Model file for the job. Use its own axes, mm. A direction names the side the tool comes from. Round coordinates to 2 decimals unless told otherwise and drop trailing zeros. Order: outer loops, then holes, each group sorted by start corner. A loop starts at its lowest first (then second) coordinate and runs counter-clockwise, first axis right, second up. Notation, with made-up numbers: M -15.5,64 L 19.5,64 A12 ccw 19.5,71 Z; hole C -17,-8.5 d10. An arc over 180 degrees is marked long. Return JSON: item names as keys, results as strings. Group by question number.
Item 1: Slice it at D-D on y = 22.5. Write the cut outline in (x, z), then the cut area to 3 significant figures.
Item 2: Which spindle directions (+Z, -Z, +X, -X, +Y, -Y) get a long thin tool onto all of the face, cutting with end or side? Do faces 5 (the face through (5.22, -2.96, 35.07)), 6 (the face through (-1, -28, 0)). Say none if no direction does.
Item 3: Probe line 1 along Y through (x, z) = (0, 27); line 2 along Y through (x, z) = (4.5, 39.5); line 3 along Z through (x, y) = (11, 0). List the from-to ranges inside material, lowest first.
Item 4: Pin check, flat tips, straight feed: pin 1 Ø5 at (y, z) = (31, 25.5) entering from -X; pin 2 Ø1.5 at (x, y) = (-12, 5.5) entering from -Z; pin 3 Ø11 at (x, y) = (3.5, -2.5) entering from -Z. Stop position of each tip, or through.
Item 5: Pull direction Y, two halves, no side cores. Call faces 1 (the face through (0, 0, 40)), 2 (the face through (-9.571, 5.423, 35.07)), 3 (the face through (-1, 1, 45)), 4 (the face through (-5.598, 42.634, 22.185)): pulls with the +Y half, pulls with the -Y half, needs draft (parallel to the pull), parting line crosses it, or undercut.
Item 6: Slice it at B-B on x = 0. Write the cut outline in (y, z), then the cut area to 3 significant figures.
Item 7: Slice it at C-C on z = 22.5. Write the cut outline in (x, y), then the cut area to 3 significant figures.
Item 8: Slice it at A-A on z = 35. Write the cut outline in (x, y).
from build123d import *

# Parameters (mm, degrees)
SKETCH1_R           = 43
SKETCH1_R_2         = 27.5
BOSS_EXTRUDE1_DEPTH = 40
SKETCH2_R           = 43
BOSS_EXTRUDE2_DEPTH = 5
BOSS_EXTRUDE3_DEPTH = 10


with BuildPart() as part:
    # Sketch1 → Boss-Extrude1 (new body)
    with BuildSketch(Plane.XY):
        Circle(SKETCH1_R)
        Circle(SKETCH1_R_2, mode=Mode.SUBTRACT)
    extrude(amount=BOSS_EXTRUDE1_DEPTH)

    # Sketch2 → Boss-Extrude2 (add)
    with BuildSketch(Plane.XY.offset(40)):
        Circle(SKETCH2_R)
    extrude(amount=BOSS_EXTRUDE2_DEPTH)

    # Sketch3 → Boss-Extrude3 (add)
    with BuildSketch(Plane(origin=(0, 0, 40), x_dir=(-1, 0, 0), z_dir=(0, 0, -1))):
        Polygon((6.350852961, 11), (-6.350852961, 11), (-12.701705922, 0), (-6.350852961, -11), (6.350852961, -11), (12.701705922, 0), align=None)
        Polygon((3.464101615, 6), (-3.464101615, 6), (-6.92820323, 0), (-3.464101615, -6), (3.464101615, -6), (6.92820323, 0), align=None, mode=Mode.SUBTRACT)
    extrude(amount=BOSS_EXTRUDE3_DEPTH)


solid = part.part
Output values:
{
 "1": {"outline": "M -36.64,0 L -15.81,0 L -15.81,40 L 15.81,40 L 15.81,0 L 36.64,0 L 36.64,45 L -36.64,45 Z", "area": "2,030 mm²"},
 "2": {"face 5": "-Z", "face 6": "-Z, +X, -X, +Y, -Y"},
 "3": {"line 1": "-43 to -27.5, 27.5 to 43", "line 2": "-42.76 to -27.13, -11 to -4.21, 4.21 to 11, 27.13 to 42.76", "line 3": "30 to 45"},
 "4": {"pin 1": "x = -32.2", "pin 2": "z = 40", "pin 3": "z = 30"},
 "5": {"face 1": "undercut", "face 2": "undercut", "face 3": "needs draft", "face 4": "parting line crosses it"},
 "6": {"outline": "M -43,0 L -27.5,0 L -27.5,40 L -11,40 L -11,30 L -6,30 L -6,40 L 6,40 L 6,30 L 11,30 L 11,40 L 27.5,40 L 27.5,0 L 43,0 L 43,45 L -43,45 Z", "area": "1,770 mm²"},
 "7": {"outline": "C 0,0 d86; hole C 0,0 d55", "area": "3,430 mm²"},
 "8": {"outline": "C 0,0 d86; M -12.7,0 L -6.35,-11 L 6.35,-11 L 12.7,0 L 6.35,11 L -6.35,11 Z; hole C 0,0 d55; hole M -6.93,0 L -3.46,-6 L 3.46,-6 L 6.93,0 L 3.46,6 L -3.46,6 Z"}
}
